Autodesk Fusion 360 part; units mm, degrees
sketch "Sketch1" plane through (0, 0, 0) normal (0, 0, 1) x (1, 0, 0)
  line L0 (-65, 20) -> (65, 20)
  line L1 (65, 20) -> (65, 0)
  line L2 (65, 0) -> (-65, 0)
  line L3 (-65, 0) -> (-65, 20)
  dimension "d1" = 130
  dimension "d2" = 20
extrude "Extrude1" add sketch "Sketch1" along normal blind 10
sketch "Sketch3" plane through (0, 0, 10) normal (0, 0, 1) x (-1, 0, 0)
  line L0 (65, -20) -> (65, 0)
  line L1 (65, -10) -> (45, -10)
  line L2 (45, -10) -> (25, -10)
  line L3 (-65, 0) -> (-65, -20)
  line L4 (-65, -10) -> (-45, -10)
  line L5 (-45, -10) -> (-25, -10)
  point P0 (65, -20)
  dimension "d10" = 20
  dimension "d11" = 20
  dimension "d12" = 20
  dimension "d13" = 20
hole "Hole1" at (-45, 10, 10) at (25, 10, 10) at (45, 10, 10) at (-25, 10, 10) direction (0, 0, -1) diameter 5.029 depth 11 tip angle 118 counterbore diameter 9.5 counterbore depth 5.5
Check sheet for the modelled part. Datum: model origin and axes. Units: mm. A direction names the side the tool comes from. Round coordinates to 2 decimals unless told otherwise and drop trailing zeros. Loops run counter-clockwise (first coordinate to the right, second up) from the corner with the lowest first, then second, coordinate; pieces in that order, holes last. Notation, with made-up numbers: M -29,20 L 0,20 A23 cw 0,40 Z; hole C 65.25,57 d6. An arc over 180 degrees is marked long. Answer as a JSON object with one key per item and string values.
1. Section check D-D (y = 10.5). State how many separate pieces and enclosed holes the cut face has, plus the area to 3 significant figures.
Reply:
{"separate pieces": "5", "enclosed holes": "0", "area": "1,000 mm²"}
2. Section check A-A (z = 7.25). Record the boundary of the cut face in (x, y).
Reply:
{"outline": "M -65,0 L 65,0 L 65,20 L -65,20 Z; hole C -45,10 d9.5; hole C -25,10 d9.5; hole C 25,10 d9.5; hole C 45,10 d9.5"}
3. Section check C-C (z = 2.5). Record the boundary of the cut face in (x, y).
Reply:
{"outline": "M -65,0 L 65,0 L 65,20 L -65,20 Z; hole C -45,10 d5.03; hole C -25,10 d5.03; hole C 25,10 d5.03; hole C 45,10 d5.03"}
4. Scan lines: line 1 (X direction, y = 10, z = 8.95); line 2 (Y direction, x = 45, z = 2.9); line 3 (X direction, y = 10, z = 1). Record each from-to range of solid material in increasing order.
Reply:
{"line 1": "x = -65 to -49.75, -40.25 to -29.75, -20.25 to 20.25, 29.75 to 40.25, 49.75 to 65", "line 2": "y = 0 to 7.49, 12.51 to 20", "line 3": "x = -65 to -47.51, -42.49 to -27.51, -22.49 to 22.49, 27.51 to 42.49, 47.51 to 65"}
5. Section check B-B (x = 45). Record the boundary of the cut face in (y, z), plus the area to 3 significant figures.
Reply:
{"outline": "M 0,0 L 7.49,0 L 7.49,4.5 L 5.25,4.5 L 5.25,10 L 0,10 Z; M 12.51,0 L 20,0 L 20,10 L 14.75,10 L 14.75,4.5 L 12.51,4.5 Z", "area": "125 mm²"}
6. Mould release check, pull along X, two halves, no side actions. Record for faces 1 (the cylindrical face through (-29.71, 10.62, 7.21)), 2 (the flat face through (-1, 20, 5)), 3 (the flat face through (-65, 10, 5)): pulls with the +X half, pulls with the -X half, needs draft (parallel to the pull), parting line crosses it, or undercut.
Reply:
{"face 1": "undercut", "face 2": "needs draft", "face 3": "pulls with the -X half"}
7. Gauge pin test, flat end, axial feed: P1, Ø5.5, axis at x = 25, y = 10, coming from the +Z side. Record the tip position at first contact, or that the pin passes through.
Reply:
{"P1": "stops at z = 4.5"}
8. Access from +Z, -Z, +X, -X, +Y, -Y to the whole of each face (thin tool, end or side, straight path). Record for faces 4 (the cylindrical face through (-49.71, 10.62, 7.21)), 5 (the cylindrical face through (22.507, 10.327, 2.218)).
Reply:
{"face 4": "+Z", "face 5": "+Z, -Z"}
